Could you check a few things on this model? Use its own coordinates, in mm. A direction names the side the tool comes from. Coordinates: 2 decimals unless noted, no trailing zeros. Order: outer loops, then holes, each group sorted by start corner. A loop starts at its lowest first (then second) coordinate and runs counter-clockwise, first axis right, second up. Notation, with made-up numbers: (-16, -38.5) - (18, -38.5) arc R20 ccw to (18, -34.5) - close; hole circle Ø9 at (1, 70). An arc over 180 degrees is marked (long way). One line per item, written item: value.
from build123d import *

# Parameters (mm, degrees)
F1_DEPTH = 25.4


with BuildPart() as f1:
    # F0 (on Top) → F1 (new body)
    with BuildSketch(Plane.XY):
        with BuildLine():
            ThreePointArc((-42.8508276872, 31.8025350571), (-41.4654203847, 11.9639712949), (-24.4785961914, 22.3049465567))
            ThreePointArc((-24.4785961914, 22.3049465567), (-25.77864226, 27.6507494196), (-29.3884073564, 31.8025350571))
            Line((-29.3884073564, 31.8025350571), (-42.8508276872, 31.8025350571))
        make_face()
        with BuildLine():
            Line((-42.8508276872, 31.8025350571), (-29.3884073564, 31.8025350571))
            ThreePointArc((-29.3884073564, 31.8025350571), (-36.1196175218, 33.945967887), (-42.8508276872, 31.8025350571))
        make_face()
        with BuildLine():
            ThreePointArc((-42.8508276872, 31.8025350571), (-36.1196175218, 33.945967887), (-29.3884073564, 31.8025350571))
            Line((-29.3884073564, 31.8025350571), (-24.0317769349, 31.8025350571))
            Line((-24.0317769349, 31.8025350571), (-24.0317769349, 38.7098751962))
            Line((-24.0317769349, 38.7098751962), (-48.207461834, 38.7098751962))
            Line((-48.207461834, 38.7098751962), (-48.207461834, 31.8025350571))
            Line((-48.207461834, 31.8025350571), (-42.8508276872, 31.8025350571))
        make_face()
    extrude(amount=F1_DEPTH)


solid = f1.part
Item 1: I want a section at D-D on x = -42. Please give me the cut outline in (y, z), then the cut area to 3 significant figures.
Conclusion:
outline: (12.26, 0) - (38.71, 0) - (38.71, 25.4) - (12.26, 25.4) - close
area: 672 mm²
Item 2: For faces 1 (the face through (-27, 31.803, 13)), 2 (the face through (-48.207, 35, 13)), which set-ups out of +Z, -Z, +X, -X, +Y, -Y let a thin tool reach every point of the face, with its end or its side?
Conclusion:
face 1: +Z, -Z, +X
face 2: +Z, -Z, -X, +Y, -Y
Item 3: I'm going to push flat-ended pins straight in: pin 1 Ø1.5 at (y, z) = (26, 12.5) entering from +X; pin 2 Ø2 at (y, z) = (21, 12) entering from -X; pin 3 Ø6 at (x, z) = (-46.5, 10.5) entering from -Y; pin 4 Ø10 at (x, y) = (-44.5, 19.5) entering from -Z. Where does each tip first touch, or does it pass through?
Conclusion:
pin 1: x = -24.86
pin 2: x = -47.76
pin 3: y = 13.3
pin 4: z = 0
Item 4: I want a section at C-C on y = 17.75. Please give me the cut outline in (x, z), then the cut area to 3 significant figures.
Conclusion:
outline: (-46.83, 0) - (-25.41, 0) - (-25.41, 25.4) - (-46.83, 25.4) - close
area: 544 mm²
Item 5: I want a section at A-A on z = 13.25. Please give me the cut outline in (x, y), then the cut area to 3 significant figures.
Conclusion:
outline: (-48.21, 31.8) - (-42.85, 31.8) arc R11.64 ccw (long way) to (-29.39, 31.8) - (-24.03, 31.8) - (-24.03, 38.71) - (-48.21, 38.71) - close
area: 573 mm²
Item 6: Thinking about a two-plate mould opening in Y: for faces 3 (the face through (-36, 38.71, 13)), 4 (the face through (-46, 31.803, 13)), 5 (the face through (-24.032, 35, 13)), which applies, pulls with the +Y half, pulls with the -Y half, needs draft (parallel to the pull), parting line crosses it, or undercut?
Conclusion:
face 3: pulls with the +Y half
face 4: undercut
face 5: needs draft
Item 7: I want a section at B-B on x = -28.5. Please give me the cut outline in (y, z), then the cut area to 3 significant figures.
Conclusion:
outline: (13.5, 0) - (31.11, 0) - (31.11, 25.4) - (13.5, 25.4) - close; (31.8, 0) - (38.71, 0) - (38.71, 25.4) - (31.8, 25.4) - close
area: 623 mm²
Item 8: If I drill on probe 1 along Y at (x, z) = (-46.75, 22.75); probe 2 along Y at (x, z) = (-26.25, 23.25); probe 3 along X at (y, z) = (20.5, 12.5), over which ranges is the centre line in solid material (lowest first)?
Conclusion:
probe 1: 17.56 to 27.05, 31.8 to 38.71
probe 2: 16.13 to 28.48, 31.8 to 38.71
probe 3: -47.62 to -24.62
